Could you check a few things on this model? Use its own coordinates, in mm. Give positions to 0.01 mm unless a question says otherwise; leave off trailing zeros. Write each loop counter-clockwise with the first axis right and the second up, starting at its lowest first coordinate (ties: lowest second). Pieces come first, ordered by that corner, then holes. Notation, with made-up numbers: (83, -9.5) - (138, -9.5) arc R27 ccw to (138, 27.5) - close; hole circle Ø9 at (50.25, 26). An arc over 180 degrees is marked (long way). Use one line per item in the form item = value.
```python
from build123d import *

# Parameters (mm, degrees)
BOSS_EXTRUDE1_DEPTH = 4
SKETCH2_R           = 2
SKETCH2_R_2         = 1.5
CUT_EXTRUDE1_DEPTH  = 4


with BuildPart() as part:
    # Sketch1 → Boss-Extrude1 (new body)
    with BuildSketch(Plane.XY):
        with BuildLine():
            Line((0, 0), (0, 45))
            Line((0, 45), (3, 45))
            Line((3, 45), (20, 0))
            ThreePointArc((20, 0), (10, -10), (0, 0))
        make_face()
    extrude(amount=BOSS_EXTRUDE1_DEPTH)

    # Sketch2 → Cut-Extrude1 (cut)
    with BuildSketch(Plane.XY.offset(4)):
        with Locations((4, 5)):
            Circle(SKETCH2_R)
        with Locations((3, 36.511049315)):
            Circle(SKETCH2_R_2)
    extrude(amount=-CUT_EXTRUDE1_DEPTH, mode=Mode.SUBTRACT)


solid = part.part
```
1. Imagine slicing it at C-C, the plane z = 0.65. List the corners of the cut face in (x, y) for me.
Response values:
outline = (0, 0) arc R10 ccw to (20, 0) - (3, 45) - (0, 45) - close; hole circle Ø3 at (3, 36.51); hole circle Ø4 at (4, 5)
2. Imagine slicing it at B-B, the plane y = 5. List the corners of the cut face in (x, z) for me.
Response values:
outline = (0, 0) - (2, 0) - (2, 4) - (0, 4) - close; (6, 0) - (18.11, 0) - (18.11, 4) - (6, 4) - close
3. For pin 1 (2 mm diameter, centred on y = 25.5, z = 1.5, fed in from -X); pin 2 (1.5 mm diameter, centred on y = 34.5, z = 3, fed in from +X), each with a flat end and sliding along its axis, tell me the tip position at first contact or that it passes through.
Response values:
pin_1 = 0
pin_2 = 7.25
4. Imagine slicing it at A-A, the plane x = 4. List the corners of the cut face in (y, z) for me.
Response values:
outline = (-8, 0) - (3, 0) - (3, 4) - (-8, 4) - close; (7, 0) - (35.39, 0) - (35.39, 4) - (7, 4) - close; (37.63, 0) - (42.35, 0) - (42.35, 4) - (37.63, 4) - close
5. If I drill on line 1 (Y direction, x = 2.25, z = 3.8); line 2 (X direction, y = 37, z = 2.85); line 3 (X direction, y = 30.5, z = 3.1), over which ranges is the centre line in solid material (lowest first)? Write a range as from..to.
Response values:
line_1 = -6.32..4.03, 5.97..35.21, 37.81..45
line_2 = 0..1.58, 4.42..6.02
line_3 = 0..8.48
6. Imagine slicing it at D-D, the plane y = 18. List the corners of the cut face in (x, z) for me, and give its area (3 significant figures).
Response values:
outline = (0, 0) - (13.2, 0) - (13.2, 4) - (0, 4) - close
area = 52.8 mm²
7. If we mould it in two halves opening along X, with no side actions, what happens to faces 1 (the face through (1, 45, 2)), 2 (the face through (2.526, 6.352, 2.028)), 3 (the face through (0, 22, 2))? For each: pulls with the +X half, pulls with the -X half, needs draft (parallel to the pull), parting line crosses it, or undercut.
Response values:
face_1 = needs draft
face_2 = undercut
face_3 = pulls with the -X half
